Could you check a few things on this model? Use its own coordinates, in mm. A direction names the side the tool comes from. Give positions to 0.01 mm unless a question says otherwise; leave off trailing zeros. Write each loop counter-clockwise with the first axis right and the second up, starting at its lowest first coordinate (ties: lowest second). Pieces come first, ordered by that corner, then holes. Notation, with made-up numbers: (-27, 23) - (-9, 23) arc R33 ccw to (-9, 54) - close; hole circle Ø3 at (-7.75, 14.5). An arc over 180 degrees is marked (long way). Use one line per item in the form item = value.
```python
from build123d import *

# Parameters (mm, degrees)
F0_R     = 1.5
F0_R_2   = 1.75
F0_R_3   = 2.75
F0_W     = 24
F0_H     = 43.8174021336
F0_W_2   = 25
F0_W_3   = 74.5545638204
F0_H_2   = 80
F1_DEPTH = 3
F2_DEPTH = 20
F3_DEPTH = 20


# Not quite as in the source:
# - a feature names something its author has since deleted; it is built from what else it names


with BuildPart() as f1:
    # F0 (on Top) → F1 (new body)
    with BuildSketch(Plane.XY):
        with BuildLine():
            ThreePointArc((-47.6736667828, -81.2138915062), (-46.0983603754, -80.2573488478), (-45.4808032601, -78.5209193664))
            ThreePointArc((-45.4808032601, -78.5209193664), (-47.6409939689, -75.8349139681), (-50.7278032601, -77.3687514099))
            Line((-50.7278032601, -77.3687514099), (-50.7278032601, -79.6730873229))
            ThreePointArc((-50.7278032601, -79.6730873229), (-49.9411999358, -80.6742988526), (-48.7879397374, -81.2138915062))
            Line((-48.7879397374, -81.2138915062), (-47.6736667828, -81.2138915062))
        make_face()
        with Locations((-48.2308032601, -78.5209193664)):
            Circle(F0_R, mode=Mode.SUBTRACT)
        with BuildLine():
            ThreePointArc((-50.7278032601, -77.3687514099), (-47.6409939689, -75.8349139681), (-45.4808032601, -78.5209193664))
            ThreePointArc((-45.4808032601, -78.5209193664), (-46.0983603754, -80.2573488478), (-47.6736667828, -81.2138915062))
            Line((-47.6736667828, -81.2138915062), (50.2721967399, -81.2138915062))
            Line((50.2721967399, -81.2138915062), (50.3258705139, 82))
            Line((50.3258705139, 82), (-42.5516068935, 82))
            Line((-42.5516068935, 82), (-42.5516068935, -17.5))
            Line((-42.5516068935, -17.5), (-50.7278032601, -23.6660409719))
            Line((-50.7278032601, -23.6660409719), (-50.7278032601, -77.3687514099))
        make_face()
        with Locations((-38.7351833579, -52.5912989332)):
            Circle(F0_R_2, mode=Mode.SUBTRACT)
        with Locations((-6.5308032601, -78.3)):
            Circle(F0_R_3, mode=Mode.SUBTRACT)
        with Locations((-23.7278032601, -52.5912989332)):
            Rectangle(F0_W, F0_H, mode=Mode.SUBTRACT)
        with Locations((-47.5, -26.9212964922)):
            Circle(F0_R_3, mode=Mode.SUBTRACT)
        with Locations((-38.9970433209, -13.3562097783)):
            Circle(F0_R_3, mode=Mode.SUBTRACT)
        with Locations((-5.8, -26.7)):
            Circle(F0_R_3, mode=Mode.SUBTRACT)
        with Locations((4.9221967399, -78.3)):
            Circle(F0_R_3, mode=Mode.SUBTRACT)
        with Locations((22.7721967399, -52.5912989332)):
            Rectangle(F0_W_2, F0_H, mode=Mode.SUBTRACT)
        with Locations((46.6221967399, -78.3)):
            Circle(F0_R_3, mode=Mode.SUBTRACT)
        with Locations((46.2721967399, -52.5912989332)):
            Circle(F0_R_2, mode=Mode.SUBTRACT)
        with Locations((5.6529477609, -26.7)):
            Circle(F0_R_3, mode=Mode.SUBTRACT)
        with Locations((47.3529477609, -26.2951753209)):
            Circle(F0_R_3, mode=Mode.SUBTRACT)
        with Locations((47.0029571713, -13.3550426021)):
            Circle(F0_R_3, mode=Mode.SUBTRACT)
        with Locations((-38.9970430732, 39.4713241122)):
            Circle(F0_R_2, mode=Mode.SUBTRACT)
        with Locations((-38.7351833579, 78.1026230454)):
            Circle(F0_R_3, mode=Mode.SUBTRACT)
        with Locations((4.2256750166, 32.5)):
            Rectangle(F0_W_3, F0_H_2, mode=Mode.SUBTRACT)
        with Locations((47.0029569268, 39.4713241122)):
            Circle(F0_R_2, mode=Mode.SUBTRACT)
        with Locations((47.2648166418, 78.1026230454)):
            Circle(F0_R_3, mode=Mode.SUBTRACT)
        with BuildLine():
            Line((-50.7278032601, -79.6730873229), (-50.7278032601, -77.3687514099))
            ThreePointArc((-50.7278032601, -77.3687514099), (-50.9808032601, -78.5209193664), (-50.7278032601, -79.6730873229))
        make_face()
        with BuildLine():
            ThreePointArc((-48.7879397374, -81.2138915062), (-48.2308032601, -81.2709193664), (-47.6736667828, -81.2138915062))
            Line((-47.6736667828, -81.2138915062), (-48.7879397374, -81.2138915062))
        make_face()
        with BuildLine():
            ThreePointArc((-48.7879397374, -81.2138915062), (-49.9411999358, -80.6742988526), (-50.7278032601, -79.6730873229))
            Line((-50.7278032601, -79.6730873229), (-50.7278032601, -81.2138915062))
            Line((-50.7278032601, -81.2138915062), (-48.7879397374, -81.2138915062))
        make_face()
    extrude(amount=F1_DEPTH)

    # F0 (on Top) → F2 (join)
    with BuildSketch(Plane.XY):
        with Locations((-38.7351833579, 78.1026230454)):
            Circle(F0_R_3)
        with Locations((-38.7351833579, 78.1026230454)):
            Circle(F0_R_2, mode=Mode.SUBTRACT)
    extrude(amount=F2_DEPTH)

    # F0 (on Top) → F3 (join)
    with BuildSketch(Plane.XY):
        with Locations((47.2648166418, 78.1026230454)):
            Circle(F0_R_3)
        with Locations((47.2648166418, 78.1026230454)):
            Circle(F0_R_2, mode=Mode.SUBTRACT)
        with Locations((-38.9970433209, -13.3562097783)):
            Circle(F0_R_3)
        with Locations((-38.9970433209, -13.3562097783)):
            Circle(F0_R_2, mode=Mode.SUBTRACT)
        with Locations((47.3529477609, -26.2951753209)):
            Circle(F0_R_3)
        with Locations((47.3529477609, -26.2951753209)):
            Circle(F0_R, mode=Mode.SUBTRACT)
        with Locations((5.6529477609, -26.7)):
            Circle(F0_R_3)
        with Locations((5.6529477609, -26.7)):
            Circle(F0_R, mode=Mode.SUBTRACT)
        with Locations((-5.8, -26.7)):
            Circle(F0_R_3)
        with Locations((-5.8, -26.7)):
            Circle(F0_R, mode=Mode.SUBTRACT)
        with Locations((-47.5, -26.9212964922)):
            Circle(F0_R_3)
        with Locations((-47.5, -26.9212964922)):
            Circle(F0_R, mode=Mode.SUBTRACT)
        with BuildLine():
            ThreePointArc((-47.6736667828, -81.2138915062), (-46.0983603754, -80.2573488478), (-45.4808032601, -78.5209193664))
            ThreePointArc((-45.4808032601, -78.5209193664), (-47.6409939689, -75.8349139681), (-50.7278032601, -77.3687514099))
            Line((-50.7278032601, -77.3687514099), (-50.7278032601, -79.6730873229))
            ThreePointArc((-50.7278032601, -79.6730873229), (-49.9411999358, -80.6742988526), (-48.7879397374, -81.2138915062))
            Line((-48.7879397374, -81.2138915062), (-47.6736667828, -81.2138915062))
        make_face()
        with Locations((-48.2308032601, -78.5209193664)):
            Circle(F0_R, mode=Mode.SUBTRACT)
        with Locations((-6.5308032601, -78.3)):
            Circle(F0_R_3)
        with Locations((-6.5308032601, -78.3)):
            Circle(F0_R, mode=Mode.SUBTRACT)
        with Locations((4.9221967399, -78.3)):
            Circle(F0_R_3)
        with Locations((4.9221967399, -78.3)):
            Circle(F0_R, mode=Mode.SUBTRACT)
        with Locations((46.6221967399, -78.3)):
            Circle(F0_R_3)
        with Locations((46.6221967399, -78.3)):
            Circle(F0_R, mode=Mode.SUBTRACT)
        with Locations((47.0029571713, -13.3550426021)):
            Circle(F0_R_3)
        with Locations((47.0029571713, -13.3550426021)):
            Circle(F0_R_2, mode=Mode.SUBTRACT)
    extrude(amount=F3_DEPTH)


solid = f1.part
```
1. Imagine slicing it at C-C, the plane y = -61.5. List the corners of the cut face in (x, z) for me.
Response values:
outline = (-50.73, 0) - (-35.73, 0) - (-35.73, 3) - (-50.73, 3) - close; (-11.73, 0) - (10.27, 0) - (10.27, 3) - (-11.73, 3) - close; (35.27, 0) - (50.28, 0) - (50.28, 3) - (35.27, 3) - close
2. If we mould it in two halves opening along Y, with no side actions, what happens to faces 4 (the face through (-39, 76, 20)), 5 (the face through (-46.58, -20.54, 1.48)), 6 (the face through (35.272, -53, 1))? For each: pulls with the +Y half, pulls with the -Y half, needs draft (parallel to the pull), parting line crosses it, or undercut.
Response values:
face_4 = needs draft
face_5 = pulls with the +Y half
face_6 = undercut
3. Which directions (+Z, -Z, +X, -X, +Y, -Y) give clear straight access to the entire face, cutting with the end or side of a thin tool? Please do faces 1 (the face through (49, -13, 20)), 2 (the face through (-6.889, -75.573, 11.381)), 3 (the face through (-24, -74.5, 1)).
Response values:
face_1 = +Z, +X, -X, +Y, -Y
face_2 = +Z
face_3 = +Z, -Z
4. For pin 1 (2 mm diameter, centred on x = 46.27, y = -52.59, fed in from -Z); pin 2 (1.5 mm diameter, centred on x = -7, z = 1.5, fed in from -Y); pin 3 (8 mm diameter, centred on y = 0.5, z = 3, fed in from +X); pin 4 (0.9 mm diameter, centred on y = -40, z = 2, fed in from -X), each with a flat end and sliding along its axis, tell me the tip position at first contact or that it passes through.
Response values:
pin_1 = through
pin_2 = -81.21
pin_3 = 50.3
pin_4 = -50.73
5. If I drill on line 1 (X direction, y = -13, z = 9); line 2 (Y direction, x = -39, z = 16.75); line 3 (Y direction, x = 11, z = 1.5), over which ranges is the centre line in solid material (lowest first)? Write a range as from..to.
Response values:
line_1 = -41.72..-40.71, -37.28..-36.27, 44.28..45.29, 48.72..49.73
line_2 = -16.11..-15.11, -11.61..-10.61, 75.37..76.37, 79.83..80.84
line_3 = -81.21..-74.5, -30.68..-7.5, 72.5..82
6. Imagine slicing it at D-D, the plane y = 29.5. List the corners of the cut face in (x, z) for me.
Response values:
outline = (-42.55, 0) - (-33.05, 0) - (-33.05, 3) - (-42.55, 3) - close; (41.5, 0) - (50.31, 0) - (50.31, 3) - (41.5, 3) - close
7. Imagine slicing it at B-B, the plane z = 16.75. State how many separate pieces and enclosed holes the cut face has, and give its area (3 significant figures).
Response values:
separate_pieces = 12
enclosed_holes = 12
area = 190 mm²
8. Imagine slicing it at A-A, the plane y = 4.5. List the corners of the cut face in (x, z) for me.
Response values:
outline = (-42.55, 0) - (-33.05, 0) - (-33.05, 3) - (-42.55, 3) - close; (41.5, 0) - (50.3, 0) - (50.3, 3) - (41.5, 3) - close
